from build123d import *

# Parameters (mm, degrees)
SKETCH1_W           = 6
SKETCH1_H           = 6
BOSS_EXTRUDE1_DEPTH = 5
CUT_EXTRUDE10_DEPTH = 12.5
CUT_EXTRUDE11_DEPTH = 2.5


with BuildPart() as part:
    # Sketch1 → Boss-Extrude1 (new body)
    with BuildSketch(Plane(origin=(0, 0, 0), x_dir=(1, 0, 0), z_dir=(0, 1, 0))):
        Rectangle(SKETCH1_W, SKETCH1_H)
    extrude(amount=BOSS_EXTRUDE1_DEPTH)

    # Sketch11 → Cut-Extrude10 (cut)
    with BuildSketch(Plane.XY.offset(3)):
        with BuildLine():
            ThreePointArc((-3, 0), (-0.780941195, 3.437129434), (3, 5))
            Line((3, 5), (-3, 5))
            Line((-3, 5), (-3, 0))
        make_face()
    extrude(amount=-CUT_EXTRUDE10_DEPTH, mode=Mode.SUBTRACT)

    # Sketch12 → Cut-Extrude11 (cut)
    with BuildSketch(Plane.XY.offset(3)):
        with BuildLine():
            Line((0, 2), (0, 4))
            ThreePointArc((0, 4), (-1.877372905, 2.283029678), (-3, 0))
            Line((-3, 0), (0, 2))
        make_face()
    extrude(amount=-CUT_EXTRUDE11_DEPTH, mode=Mode.SUBTRACT)


solid = part.part
Verification items for the finished model (mm, model axes). A direction names the side the tool comes from. Give positions to 0.01 mm unless a question says otherwise; leave off trailing zeros. Loops run counter-clockwise (first coordinate to the right, second up) from the corner with the lowest first, then second, coordinate; pieces in that order, holes last.
1. Cross-section at A-A on z = 1.1. Record the cut outline in (x, y), and give its area (3 significant figures).
Derived:
outline: (-3, 0) - (3, 0) - (3, 5) arc R6.86 ccw to (0, 4) - (0, 2) - close
area: 16.9 mm2
2. Cross-section at C-C on x = -1.75. Record the cut outline in (y, z), and give its area (3 significant figures).
Derived:
outline: (0, -3) - (2.45, -3) - (2.45, 0.5) - (0.83, 0.5) - (0.83, 3) - (0, 3) - close
area: 10.6 mm2
3. Material ranges on probe 1 along Z at (x, y) = (-0.75, 2.8); probe 2 along X at (y, z) = (3.8, 1.25); probe 3 along Y at (x, z) = (0.25, -0.45), recorded low to high.
Derived:
probe 1: z = -3 to 0.5
probe 2: x = 0 to 3
probe 3: y = 0 to 4.15
4. Cross-section at D-D on z = -2.2. Record the cut outline in (x, y).
Derived:
outline: (-3, 0) - (3, 0) - (3, 5) arc R6.86 ccw to start
5. Release check for a two-part mould opening along Y. For faces 3 (the flat face through (-1.5, 1, 1.8)), 4 (the flat face through (0, 0, 0)), 5 (the flat face through (0, 3, 2)) record: +Y half, -Y half, draft (parallel to the pull), parting line (faces both ways), or undercut.
Derived:
face 3: +Y half
face 4: -Y half
face 5: draft
6. Tool access check on faces 1 (the flat face through (1, 2, -3)), 2 (the flat face through (-1, 2, 0.5)). Record the directions out of +Z, -Z, +X, -X, +Y, -Y that give a thin tool (end or side, any length) a straight path to the whole face; none if there is none.
Derived:
face 1: -Z, +X, -X, +Y, -Y
face 2: +Z, -X, +Y
7. Go/stop test with flat-tipped pins: P1, Ø1, axis at y = 3, z = 2.5, coming from the -X side; P2, Ø2, axis at x = -2, z = 1, coming from the +Y side; P3, Ø1.5, axis at x = -1.5, y = 2, coming from the +Z side. Record where each tip stops, or that it passes through.
Derived:
P1: stops at x = 0
P2: stops at y = 3.12
P3: stops at z = 0.5
8. Cross-section at B-B on y = 0.75. Record the cut outline in (x, z) (3 decimals).
Derived:
outline: (-2.745, -3) - (3, -3) - (3, 3) - (-1.875, 3) - (-1.875, 0.5) - (-2.745, 0.5) - close
